Here's how the part is built. I have some questions about the finished solid (model axes, mm). Face numbers are marked on the shaded views. A direction names the side the tool comes from. Round coordinates to 2 decimals unless told otherwise and drop trailing zeros. Write each loop counter-clockwise with the first axis right and the second up, starting at its lowest first coordinate (ties: lowest second). Pieces come first, ordered by that corner, then holes. Notation, with made-up numbers: M 18,19 L 45,19 A33 cw 45,52 Z; hole C 50,-10.75 d4. An arc over 180 degrees is marked long. Use one line per item in the form item = value. Start each with the question number.
Q1. I need wall thicknesses on line 1 along Y through (x, z) = (0, 0.4); line 2 along Y through (x, z) = (-0.5, -0.95); line 3 along X through (y, z) = (94, 1.15). Which ranges of each line are inside material? Lowest first, please. Write a range as from..to.
Q2. I want a section at B-B on x = -12.5. List the corners of the cut face in (y, z) for me.
Q3. For the marked faces 1 and 2, which set-ups out of +Z, -Z, +X, -X, +Y, -Y let a thin tool reach every point of the face, with its end or its side?
Q4. I'm going to push flat-ended pins straight in: pin 1 Ø8 at (x, y) = (0.5, 88) entering from +Z; pin 2 Ø1.5 at (x, z) = (9, 1) entering from -Y; pin 3 Ø0.5 at (x, z) = (-4.5, -0.5) entering from -Y. Where does each tip first touch, or does it pass through?
Q5. I want a section at D-D on x = -27. List the corners of the cut face in (y, z) for me, and give its area (3 significant figures).
Q6. I want a section at C-C on y = 48. List the corners of the cut face in (x, z) for me.
Q7. I want a section at A-A on y = 0. List the corners of the cut face in (x, z) for me, and give its area (3 significant figures).
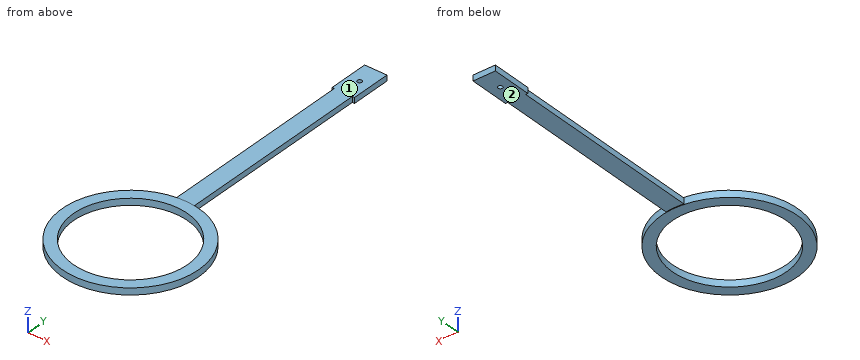
```python
from build123d import *

# Parameters (mm, degrees)
SKETCH1_R           = 30.5
BOSS_EXTRUDE1_DEPTH = 1.5
SKETCH2_W           = 8
SKETCH2_H           = 93
BOSS_EXTRUDE2_DEPTH = 1.25
SKETCH3_W           = 10
SKETCH3_H           = 18
BOSS_EXTRUDE3_DEPTH = 1.25
SKETCH4_R           = 25.5
CUT_EXTRUDE1_DEPTH  = 10
SKETCH5_R           = 1
CUT_EXTRUDE2_DEPTH  = 10


with BuildPart() as part:
    # Sketch1 → Boss-Extrude1 (new, symmetric)
    with BuildSketch(Plane.XY):
        Circle(SKETCH1_R)
    extrude(amount=BOSS_EXTRUDE1_DEPTH, both=True)

    # Sketch2 → Boss-Extrude2 (add, symmetric)
    with BuildSketch(Plane.XY):
        with Locations((0, 71.5)):
            Rectangle(SKETCH2_W, SKETCH2_H)
    extrude(amount=BOSS_EXTRUDE2_DEPTH, both=True)

    # Sketch3 → Boss-Extrude3 (add, symmetric)
    with BuildSketch(Plane.XY):
        with Locations((0, 127)):
            Rectangle(SKETCH3_W, SKETCH3_H)
    extrude(amount=BOSS_EXTRUDE3_DEPTH, both=True)

    # Sketch4 → Cut-Extrude1 (cut, symmetric)
    with BuildSketch(Plane.XY):
        Circle(SKETCH4_R)
    extrude(amount=CUT_EXTRUDE1_DEPTH, both=True, mode=Mode.SUBTRACT)

    # Sketch5 → Cut-Extrude2 (cut, symmetric)
    with BuildSketch(Plane.XY):
        with Locations((0, 127)):
            Circle(SKETCH5_R)
    extrude(amount=CUT_EXTRUDE2_DEPTH, both=True, mode=Mode.SUBTRACT)


solid = part.part
```
Reported:
q1.line_1 = -30.5..-25.5, 25.5..126, 128..136
q1.line_2 = -30.5..-25.5, 25.5..126.13, 127.87..136
q1.line_3 = -4..4
q2.outline = M -27.82,-1.5 L -22.23,-1.5 L -22.23,1.5 L -27.82,1.5 Z; M 22.23,-1.5 L 27.82,-1.5 L 27.82,1.5 L 22.23,1.5 Z
q3.face_1 = +Z, +X, -X, +Y
q3.face_2 = -Z, +X, -X, +Y
q4.pin_1 = 1.25
q4.pin_2 = -29.36
q4.pin_3 = -30.2
q5.outline = M -14.19,-1.5 L 14.19,-1.5 L 14.19,1.5 L -14.19,1.5 Z
q5.area = 85.1 mm^2
q6.outline = M -4,-1.25 L 4,-1.25 L 4,1.25 L -4,1.25 Z
q7.outline = M -30.5,-1.5 L -25.5,-1.5 L -25.5,1.5 L -30.5,1.5 Z; M 25.5,-1.5 L 30.5,-1.5 L 30.5,1.5 L 25.5,1.5 Z
q7.area = 30.0 mm^2
